Autodesk Inventor part; units mm, degrees
ref_plane "YZ Plane" through (0, 0, 0) normal (1, 0, 0) x (0, 1, 0)
ref_plane "XZ Plane" through (0, 0, 0) normal (0, 1, 0) x (-1, 0, 0)
ref_plane "XY Plane" through (0, 0, 0) normal (0, 0, 1) x (1, 0, 0)
sketch "Sketch1" plane through (0, 0, 0) normal (0, 0, 1) x (1, 0, 0)
  line L0 (-75, -60) -> (75, -60)
  line L1 (75, -60) -> (75, 60)
  line L2 (75, 60) -> (-75, 60)
  line L3 (-75, 60) -> (-75, -60)
  line L4 (-75, -60) -> (75, 60) construction
  line L5 (75, -60) -> (-75, 60) construction
  circle A0 centre (-55, 40) radius 8
  circle A1 centre (-55, -40) radius 8
  circle A2 centre (55, 40) radius 8
  circle A3 centre (55, -40) radius 8
  line L6 (0, 60) -> (0, -60) construction
  line L7 (-75, 0) -> (75, 0) construction
  point P0 (0, 0)
  dimension "d154" = 150
  dimension "d155" = 120
  dimension "d157" = 20
  dimension "d158" = 20
  dimension "d159" = 16
extrude "Plate5" add sketch "Sketch1" along normal blind 6 contours L3 L2 L1 L0 | A0 | A2
fillet "Corner Round1" radius 6 4 edges at (-75, -60, 3) (75, -60, 3) (75, 60, 3) (-75, 60, 3)
properties part number "NDM-VOS pillar 2 plate 1" material "Steel"
Can you work these out from the model? Positions are in its coordinate system, mm. Give positions to 0.01 mm unless a question says otherwise; leave off trailing zeros. Loops run counter-clockwise (first coordinate to the right, second up) from the corner with the lowest first, then second, coordinate; pieces in that order, holes last. Notation, with made-up numbers: (48.25, -32) - (60.25, -32) arc R22 cw to (60.25, 5) - close; hole circle Ø3 at (85, 78.25). An arc over 180 degrees is marked (long way). Return JSON: item names as keys, results as strings.
1. If I drill on line 1 (Y direction, x = -55, z = 1.9); line 2 (X direction, y = -41, z = 4.5); line 3 (X direction, y = -34, z = 2.3), over which ranges is the centre line in solid material (lowest first)?
Output values:
{"line 1": "y = -60 to -48, -32 to 60", "line 2": "x = -75 to -62.94, -47.06 to 47.06, 62.94 to 75", "line 3": "x = -75 to -60.29, -49.71 to 49.71, 60.29 to 75"}
2. We'd pull the mould along Y, two halves only. Please class faces 1 (the face through (-75, 1, 3)), 2 (the face through (-73.196, 58.289, 3.042)), 3 (the face through (49.1, -45.4, 3)), 4 (the face through (-73.289, -58.196, 3.042)): +Y half, -Y half, draft (parallel to the pull), parting line (faces both ways), or undercut.
Output values:
{"face 1": "draft", "face 2": "+Y half", "face 3": "undercut", "face 4": "-Y half"}
3. I want a section at A-A on x = -55. Please give me the cut outline in (y, z), and give its area (3 significant figures).
Output values:
{"outline": "(-60, 0) - (-48, 0) - (-48, 6) - (-60, 6) - close; (-32, 0) - (60, 0) - (60, 6) - (-32, 6) - close", "area": "624 mm²"}
4. I want a section at B-B on y = -40. Please give me the cut outline in (x, z), and give its area (3 significant figures).
Output values:
{"outline": "(-75, 0) - (-63, 0) - (-63, 6) - (-75, 6) - close; (-47, 0) - (47, 0) - (47, 6) - (-47, 6) - close; (63, 0) - (75, 0) - (75, 6) - (63, 6) - close", "area": "708 mm²"}
5. I want a section at D-D on x = 53.5. Please give me the cut outline in (y, z), and give its area (3 significant figures).
Output values:
{"outline": "(-60, 0) - (-47.86, 0) - (-47.86, 6) - (-60, 6) - close; (-32.14, 0) - (60, 0) - (60, 6) - (-32.14, 6) - close", "area": "626 mm²"}
6. I want a section at C-C on z = 2.1. Please give me the cut outline in (x, y).
Output values:
{"outline": "(-75, -54) arc R6 ccw to (-69, -60) - (69, -60) arc R6 ccw to (75, -54) - (75, 54) arc R6 ccw to (69, 60) - (-69, 60) arc R6 ccw to (-75, 54) - close; hole circle Ø16 at (-55, -40); hole circle Ø16 at (55, -40)"}
